Geometry check sheet. Reference: the model listing, model coordinates, mm. Coordinates: 2 decimals unless noted, no trailing zeros. Loops run counter-clockwise (first coordinate to the right, second up) from the corner with the lowest first, then second, coordinate; pieces in that order, holes last.
from build123d import *

# Parameters (mm, degrees)
F0_R     = 40
F1_DEPTH = 56
F2_D     = 8
F3_R     = 2


with BuildPart() as f1:
    # F0 (on Top) → F1 (new body)
    with BuildSketch(Plane.XY):
        Circle(F0_R)
    extrude(amount=F1_DEPTH)

    # F2 (through all)
    with Locations(Plane(origin=(0, 0, 0), x_dir=(1, 0, 0), z_dir=(0, 0, -1))):
        with Locations((0, 0)):
            Hole(F2_D / 2)

    # F3
    f3_edges = [f1.edges().sort_by_distance(p)[0] for p in [
        (40, 0, 28),
        (-40, 0, 0),
        (-40, 0, 56),
    ]]
    fillet(f3_edges, radius=F3_R)


solid = f1.part
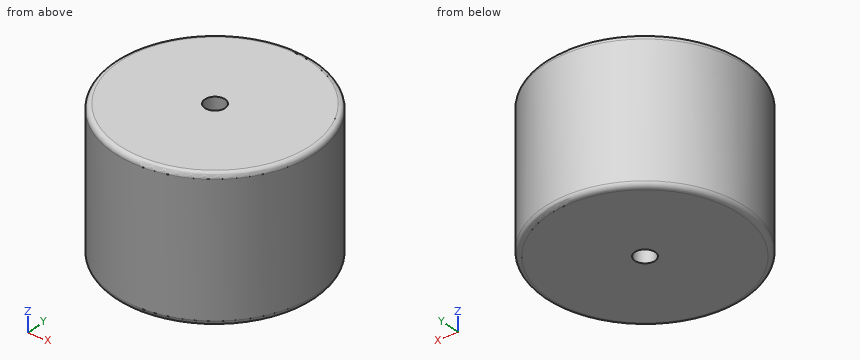
1) Section check A-A on y = 0. Record the cut outline in (x, z).
Data:
outline: (-40, 2) arc R2 ccw to (-38, 0) - (-4, 0) - (-4, 56) - (-38, 56) arc R2 ccw to (-40, 54) - close; (4, 0) - (38, 0) arc R2 ccw to (40, 2) - (40, 54) arc R2 ccw to (38, 56) - (4, 56) - close
2) Section check C-C on z = 9.5. Record the cut outline in (x, y), and give its area (3 significant figures).
Data:
outline: circle Ø80 at (0, 0); hole circle Ø8 at (0, 0)
area: 4,980 mm2
3) Depth check by flat-ended pin: pin 1 (8 mm diameter, centred on y = 7.5, z = 47, fed in from -X); pin 2 (12 mm diameter, centred on x = -9.5, z = 42.5, fed in from +Y); pin 3 (12 mm diameter, centred on y = 30, z = 21.5, fed in from +X); pin 4 (9 mm diameter, centred on x = 0, y = 0, fed in from -Z). Enter the tip coordinate at first touch or a pass-through.
Data:
pin 1: stops at x = -39.85
pin 2: stops at y = 39.85
pin 3: stops at x = 32
pin 4: stops at z = 0
4) Material ranges on probe 1 along Y at (x, z) = (0, 20.5); probe 2 along X at (y, z) = (3, 24); probe 3 along X at (y, z) = (-37, 45), recorded low to high.
Data:
probe 1: y = -40 to -4, 4 to 40
probe 2: x = -39.89 to -2.65, 2.65 to 39.89
probe 3: x = -15.2 to 15.2
